Design review of the part built by this model. Coordinates are the model's own, in mm. Face numbers are marked on the shaded views. A direction names the side the tool comes from. Round coordinates to 2 decimals unless told otherwise and drop trailing zeros. Order: outer loops, then holes, each group sorted by start corner. A loop starts at its lowest first (then second) coordinate and runs counter-clockwise, first axis right, second up. Notation, with made-up numbers: (43, -39.5) - (80, -39.5) arc R18 cw to (80, -26.5) - close; hole circle Ø3 at (21, 29.5). An arc over 180 degrees is marked (long way). Use CSV: the item, a comma, the result in double quotes. Start each with the question number.
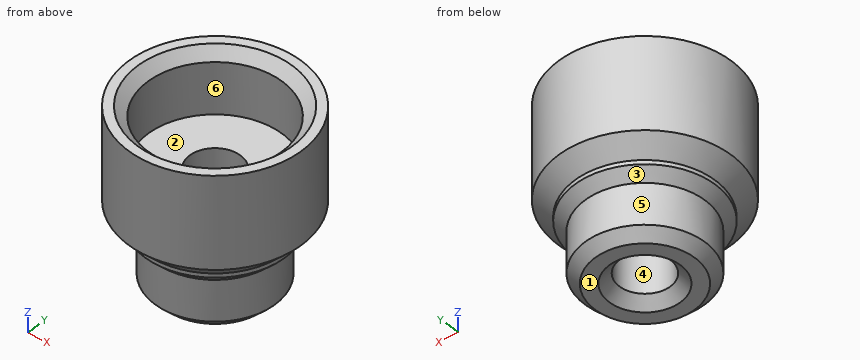
from build123d import *

# Parameters (mm, degrees)
SKETCH1_R           = 2.95
SKETCH1_R_2         = 1.25
BOSS_EXTRUDE1_DEPTH = 3
SKETCH2_R           = 4.25
SKETCH2_R_2         = 1.25
BOSS_EXTRUDE2_DEPTH = 5.5
SKETCH3_R           = 3.3
CUT_EXTRUDE1_DEPTH  = 3
CHAMFER1_SIZE       = 0.5
CHAMFER2_SIZE       = 0.5
BOSS_EXTRUDE3_START = 0.5
SKETCH4_R           = 3.45
SKETCH4_R_2         = 1.25
BOSS_EXTRUDE3_DEPTH = 0.5
CHAMFER3_SIZE       = 1
CHAMFER4_SIZE       = 0.5
CHAMFER6_SIZE       = 0.5


# Some blends are built 0.0001 mm under size
with BuildPart() as part:
    # Sketch1 → Boss-Extrude1 (new body)
    with BuildSketch(Plane.XY):
        Circle(SKETCH1_R)
        Circle(SKETCH1_R_2, mode=Mode.SUBTRACT)
    extrude(amount=BOSS_EXTRUDE1_DEPTH)

    # Sketch2 → Boss-Extrude2 (add)
    with BuildSketch(Plane.XY.offset(3)):
        Circle(SKETCH2_R)
        Circle(SKETCH2_R_2, mode=Mode.SUBTRACT)
    extrude(amount=BOSS_EXTRUDE2_DEPTH)

    # Sketch3 → Cut-Extrude1 (cut)
    with BuildSketch(Plane.XY.offset(8.5)):
        Circle(SKETCH3_R)
    extrude(amount=-CUT_EXTRUDE1_DEPTH, mode=Mode.SUBTRACT)

    # Chamfer1
    chamfer1_edges = [part.edges().sort_by_distance(p)[0] for p in [
        (-3.3, 0, 8.5),
    ]]
    chamfer(chamfer1_edges, length=CHAMFER1_SIZE)

    # Chamfer2
    chamfer2_edges = [part.edges().sort_by_distance(p)[0] for p in [
        (-2.95, 0, 0),
    ]]
    chamfer(chamfer2_edges, length=CHAMFER2_SIZE)

    # Sketch4 → Boss-Extrude3 (add)
    with BuildSketch(Plane(origin=(0, 0, 3), x_dir=(-1, 0, 0), z_dir=(0, 0, -1)).offset(BOSS_EXTRUDE3_START)):
        with Locations(Location((0, 0, 0), (0, 0, 180))):
            Circle(SKETCH4_R)
        with Locations(Location((0, 0, 0), (0, 0, 180))):
            Circle(SKETCH4_R_2, mode=Mode.SUBTRACT)
    extrude(amount=-BOSS_EXTRUDE3_DEPTH)

    # Chamfer3
    # the kernel refuses this chamfer: 1 mm, written as the material it takes off along each edge
    with BuildSketch(Plane(origin=(0, 0, 3), x_dir=(1, 0, 0), z_dir=(0, -1, 0))) as chamfer3_piece_1_section:
        Polygon((4.25 - CHAMFER3_SIZE, 0), (4.25, CHAMFER3_SIZE), (4.25, 0), align=None)
    chamfer3_piece_1 = revolve(axis=Axis((0, 0, 3), (0, 0, 1)), mode=Mode.PRIVATE)
    chamfer3_piece_1 = chamfer3_piece_1 - Plane(origin=(0, 0, 3.597538835), x_dir=(1, 0, 0), z_dir=(0, 0, -1)) * Cylinder(3.45, 17, mode=Mode.PRIVATE)
    add(chamfer3_piece_1, mode=Mode.SUBTRACT)

    # Chamfer4
    chamfer4_edges = [part.edges().sort_by_distance(p)[0] for p in [
        (-1.25, 0, 0),
    ]]
    chamfer(chamfer4_edges, length=CHAMFER4_SIZE)

    # Chamfer6
    chamfer6_edges = [part.edges().sort_by_distance(p)[0] for p in [
        (-3.45, 0, 2.5),
    ]]
    chamfer(chamfer6_edges, length=CHAMFER6_SIZE - 0.0001)  # a hair under: the kernel refuses the full size


solid = part.part
Q1. Clearance check with flat-ended pins moving along their axes: pin 1 (3 mm diameter, centred on x = 0, y = 0, fed in from -Z); pin 2 (1.5 mm diameter, centred on x = -2.5, z = 5, fed in from +Y); pin 3 (2 mm diameter, centred on y = -3, z = 4, fed in from -X). State where each tip first meets the part, or that it passes through.
Q2. Tool access review of the marked faces 4, 5 and 6: name each direction out of +Z, -Z, +X, -X, +Y, -Y from which nothing blocks a thin tool from reaching the whole face with its end or side.
Q3. Take a section at D-D (z = 8.25). State the section outline as (x, y) points.
Q4. The part is to be moulded in two halves that separate along X. For the marked faces 1, 2 and 3, say which applies: +X half, -X half, draft (parallel to the pull), parting line (faces both ways), or undercut.
Q5. Take a section at C-C (z = 3.5). State the section outline as (x, y) points, plus the area to 3 significant figures.
Q6. For L1, parallel to X at y = 0, z = 1.65; L2, parallel to Y at x = 0, z = 6.5; L3, parallel to Y at x = -0.75, z = 3.75, list the stretches that pass through material, from the lowest coordinate up. Write a range as [from, to].
Findings below:
1,pin 1,"stops at z = 0.25"
1,pin 2,"stops at y = 3.87"
1,pin 3,"stops at x = -3.75"
2,face 4,"+Z, -Z"
2,face 5,"-Z"
2,face 6,"+Z"
3,outline,"circle Ø8.5 at (0, 0); hole circle Ø7.1 at (0, 0)"
4,face 1,"draft"
4,face 2,"undercut"
4,face 3,"parting line"
5,outline,"circle Ø7.5 at (0, 0); hole circle Ø2.5 at (0, 0)"
5,area,"39.3 mm^2"
6,L1,"x = [-2.95, -1.25], [1.25, 2.95]"
6,L2,"y = [-4.25, -3.3], [3.3, 4.25]"
6,L3,"y = [-3.93, -1], [1, 3.93]"
